Source: three-view drawing plus pictorial views. Frame: mm from the lowest corner of the part. A direction names the side the tool comes from. Coordinates: 2 decimals unless noted, no trailing zeros. Loops run counter-clockwise (first coordinate to the right, second up) from the corner with the lowest first, then second, coordinate; pieces in that order, holes last. Notation, with made-up numbers: M 24,23.25 L 69,23.25 A32 ccw 69,50.25 Z; hole C 6,7 d1. An arc over 180 degrees is marked long. Use a Markdown table: item, result. Add a question column.
1. Set-up query: the marked faces 1 and 2. Return all of +Z, -Z, +X, -X, +Y, -Y with unobstructed straight access to the full face (end or side cutting, diameter ignored); none if empty.
2. Line query: L1, parallel to X at y = 7, z = 2.7; L2, parallel to X at y = 1.15, z = 2.7; L3, parallel to Y at x = 3.65, z = 5.1. Output: solid intervals per line, ascending. Write a range as [from, to].
3. Draft query along Z for the marked faces 3, 4 and 5. Return one class per face: +Z half, -Z half, draft (parallel to the pull), parting line (faces both ways), or undercut.
4. Section D-D on y = 19.25. Output: boundary loops of the cut face in (x, z), then the cut area to 3 significant figures.
5. Pin query (flat end, axial travel): pin 1 (1.5 mm diameter, centred on x = 2, z = 2, fed in from -Y); pin 2 (1 mm diameter, centred on x = 1, y = 18, fed in from +Z); pin 3 (1.2 mm diameter, centred on x = 2.5, z = 2.5, fed in from -Y); pin 4 (0.5 mm diameter, centred on x = 2.5, z = 3, fed in from -Y). Return the tip coordinate at first contact, or that it passes through.
6. Section C-C on y = 5.75. Output: boundary loops of the cut face in (x, z), then the cut area to 3 significant figures.
7. Section A-A on x = 2.7. Output: boundary loops of the cut face in (y, z).
8. Section B-B on z = 2.7. Output: boundary loops of the cut face in (x, y), then the cut area to 3 significant figures.
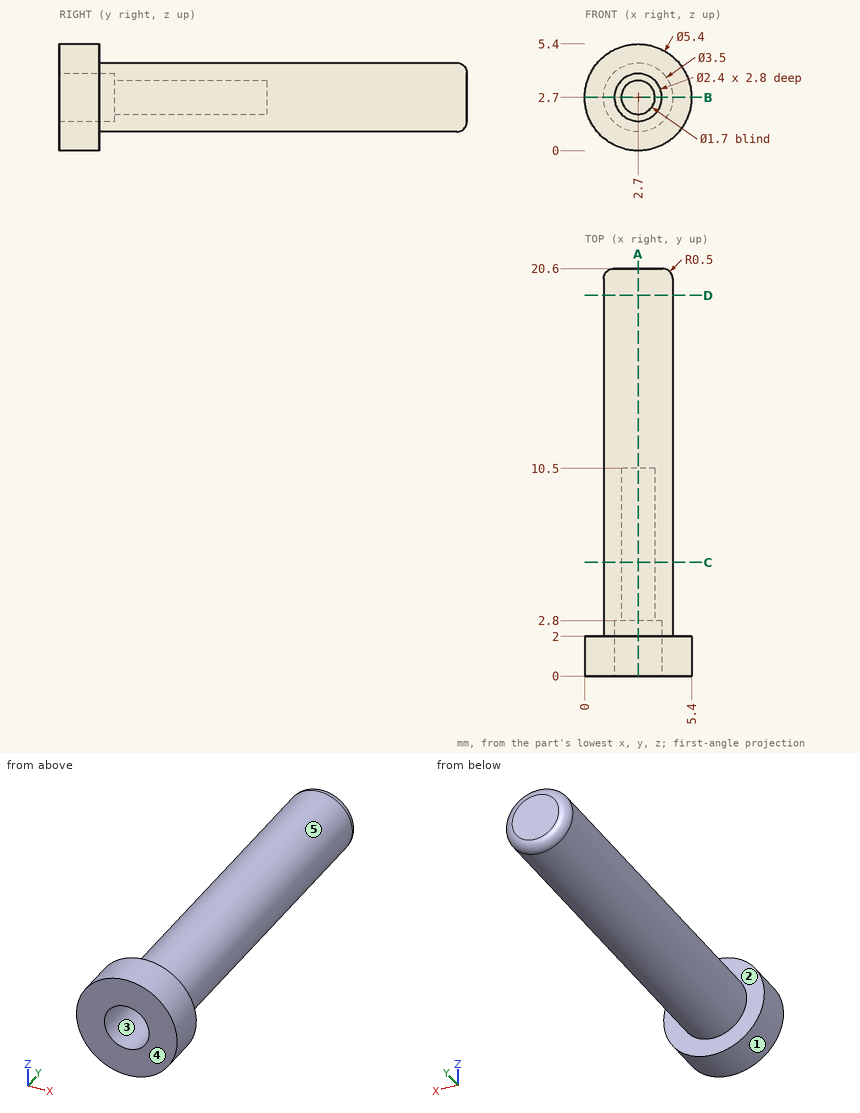
Answers below:
| question | item | result |
|---|---|---|
| 1 | face 1 | +Y, -Y |
| 1 | face 2 | +Y |
| 2 | L1 | x = [0.95, 1.85], [3.55, 4.45] |
| 2 | L2 | x = [0, 1.5], [3.9, 5.4] |
| 2 | L3 | y = [0, 2] |
| 3 | face 3 | undercut |
| 3 | face 4 | draft |
| 3 | face 5 | parting line |
| 4 | outline | C 2.7,2.7 d3.5 |
| 4 | area | 9.62 mm² |
| 5 | pin 1 | stops at y = 0 |
| 5 | pin 2 | stops at z = 3.97 |
| 5 | pin 3 | stops at y = 2.8 |
| 5 | pin 4 | stops at y = 10.5 |
| 6 | outline | C 2.7,2.7 d3.5; hole C 2.7,2.7 d1.7 |
| 6 | area | 7.35 mm² |
| 7 | outline | M 0,0 L 2,0 L 2,0.95 L 20.1,0.95 A0.5 ccw 20.6,1.45 L 20.6,3.95 A0.5 ccw 20.1,4.45 L 2,4.45 L 2,5.4 L 0,5.4 L 0,3.9 L 2.8,3.9 L 2.8,3.55 L 10.5,3.55 L 10.5,1.85 L 2.8,1.85 L 2.8,1.5 L 0,1.5 Z |
| 8 | outline | M 0,0 L 1.5,0 L 1.5,2.8 L 1.85,2.8 L 1.85,10.5 L 3.55,10.5 L 3.55,2.8 L 3.9,2.8 L 3.9,0 L 5.4,0 L 5.4,2 L 4.45,2 L 4.45,20.1 A0.5 ccw 3.95,20.6 L 1.45,20.6 A0.5 ccw 0.95,20.1 L 0.95,2 L 0,2 Z |
| 8 | area | 56.0 mm² |
